from build123d import *

# Parameters (mm, degrees)
SKETCH_1_R          = 1.7
EXTRUDE_1_DEPTH     = 4
SKETCH_2_R          = 1.5
SKETCH_2_R_2        = 2
CUT_EXTRUDE_1_DEPTH = 71.292247083
FILLET_1_R          = 5
FILLET_2_R          = 3


with BuildPart() as part:
    # 草图1 → 凸台-拉伸1 (new body)
    with BuildSketch(Plane(origin=(0, 0, 0), x_dir=(1, 0, 0), z_dir=(0, 1, 0))):
        Polygon((0, 0), (0, 30), (39, 30), (39, 38), (59, 38), (59, -38), (39, -38), (39, -30), (0, -30), align=None)
        with Locations(Location((42.5, 25, 0), (0, 0, 270))):
            Circle(SKETCH_1_R, mode=Mode.SUBTRACT)
        with Locations(Location((42.5, -25, 0), (0, 0, 270))):
            Circle(SKETCH_1_R, mode=Mode.SUBTRACT)
        with Locations(Location((42.5, 0, 0), (0, 0, 270))):
            Circle(SKETCH_1_R, mode=Mode.SUBTRACT)
        with Locations(Location((53, 30, 0), (0, 0, 270))):
            Circle(SKETCH_1_R, mode=Mode.SUBTRACT)
        with Locations(Location((53, 0, 0), (0, 0, 270))):
            Circle(SKETCH_1_R, mode=Mode.SUBTRACT)
        with Locations(Location((53, -30, 0), (0, 0, 270))):
            Circle(SKETCH_1_R, mode=Mode.SUBTRACT)
    extrude(amount=EXTRUDE_1_DEPTH)

    # 草图2 → 切除-拉伸1 (cut, through all)
    with BuildSketch(Plane(origin=(0, 4, 0), x_dir=(1, 0, 0), z_dir=(0, 1, 0))):
        with Locations(Location((32.5, 0.5, 0), (0, 0, 270))):
            Circle(SKETCH_2_R)
        with Locations(Location((5, 0.5, 0), (0, 0, 270))):
            Circle(SKETCH_2_R_2)
        with Locations(Location((5, 10.5, 0), (0, 0, 270))):
            Circle(SKETCH_2_R_2)
        with Locations(Location((53, 10.5, 0), (0, 0, 270))):
            Circle(SKETCH_2_R_2)
        with Locations(Location((29, 18, 0), (0, 0, 270))):
            Circle(SKETCH_2_R)
        with Locations(Location((18.5, -6.5, 0), (0, 0, 270))):
            Circle(SKETCH_2_R)
        with Locations(Location((11.5, 0.5, 0), (0, 0, 270))):
            Circle(SKETCH_2_R)
        with Locations(Location((25.5, 0.5, 0), (0, 0, 270))):
            Circle(SKETCH_2_R)
        with Locations(Location((18.5, 7.5, 0), (0, 0, 270))):
            Circle(SKETCH_2_R)
    extrude(amount=-CUT_EXTRUDE_1_DEPTH, mode=Mode.SUBTRACT)

    # 圆角1
    fillet_1_edges = [part.edges().sort_by_distance(p)[0] for p in [
        (59, 2, 38),
        (39, 2, 30),
        (0, 2, 30),
        (0, 2, -30),
        (39, 2, -30),
        (59, 2, -38),
    ]]
    fillet(fillet_1_edges, radius=FILLET_1_R)

    # 圆角2
    fillet_2_edges = [part.edges().sort_by_distance(p)[0] for p in [
        (39, 2, 38),
        (39, 2, -38),
    ]]
    fillet(fillet_2_edges, radius=FILLET_2_R - 0.0001)  # a hair under: the kernel refuses the full size


solid = part.part
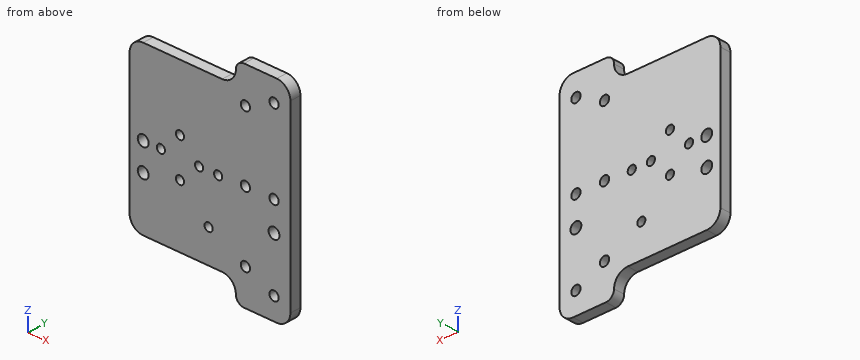
The model under review builds one solid part; all positions refer to its coordinate system, in mm. Coordinates: 2 decimals unless noted, no trailing zeros. Loops run counter-clockwise (first coordinate to the right, second up) from the corner with the lowest first, then second, coordinate; pieces in that order, holes last.
(1) Consider section C-C, the plane y = 1.1. Give the number of separate pieces and of enclosed holes in the cut face, plus the area to 3 significant figures.
Determined:
separate pieces: 1
enclosed holes: 15
area: 3,710 mm2
(2) Consider section D-D, the plane x = 53. Give the boundary of the cut face in (y, z), plus the area to 3 significant figures.
Determined:
outline: (0, -38) - (4, -38) - (4, -31.7) - (0, -31.7) - close; (0, -28.3) - (4, -28.3) - (4, -12.5) - (0, -12.5) - close; (0, -8.5) - (4, -8.5) - (4, -1.7) - (0, -1.7) - close; (0, 1.7) - (4, 1.7) - (4, 28.3) - (0, 28.3) - close; (0, 31.7) - (4, 31.7) - (4, 38) - (0, 38) - close
area: 247 mm2
(3) Wall thickness on L1, parallel to X at y = 2.05, z = -10.5; L2, parallel to Z at x = 19, y = 2.25; L3, parallel to Z at x = 14.5, y = 3.7: over which ranges is each line inside the solid? List them lowest first.
Determined:
L1: x = 0 to 3, 7 to 51, 55 to 59
L2: z = -30 to -8.91, -6.09 to 5.09, 7.91 to 30
L3: z = -30 to 30
(4) Consider section B-B, the plane z = -10.5. Give the boundary of the cut face in (x, y).
Determined:
outline: (0, 0) - (3, 0) - (3, 4) - (0, 4) - close; (7, 0) - (51, 0) - (51, 4) - (7, 4) - close; (55, 0) - (59, 0) - (59, 4) - (55, 4) - close
(5) Insertion check: P1, Ø3, axis at x = 53, z = -30, coming from the -Y side. The pin has a flat end and moves straight along its axis. Give the tip position at first contact, or say it passes through.
Determined:
P1: passes through
(6) Consider section A-A, the plane x = 25.5. Give the boundary of the cut face in (y, z), plus the area to 3 significant figures.
Determined:
outline: (0, -30) - (4, -30) - (4, -2) - (0, -2) - close; (0, 1) - (4, 1) - (4, 30) - (0, 30) - close
area: 228 mm2
